Can you work these out from the model? Positions are in its coordinate system, mm. Face numbers are marked on the shaded views. A direction names the side the tool comes from. Coordinates: 2 decimals unless noted, no trailing zeros. Order: outer loops, then holes, each group sorted by start corner. A loop starts at its lowest first (then second) coordinate and runs counter-clockwise, first axis right, second up. Notation, with made-up numbers: (-6, -38.5) -> (14, -38.5) arc R18 cw to (14, -30.5) -> close; hole circle Ø7 at (62, 86.5). An arc over 180 degrees is marked (long way). Answer in a Markdown table with one row per item.
```python
from build123d import *

# Parameters (mm, degrees)
F0_W           = 50
F0_H           = 46
F0_R           = 11
F1_DEPTH       = 20
F2_W           = 44
F2_H           = 43
F3_DEPTH       = 17
F4_SIZE2       = 17
F4_SIZE        = 42
F5_D           = 3.1
F5_CSINK_D     = 6.72
F5_CSINK_ANGLE = 90
F6_T1_DEPTH    = 23.5734639037
F7_SIZE        = 1.5
F9_D           = 4.1
F9_CSINK_D     = 9
F9_CSINK_ANGLE = 90


# Not quite as in the source:
# - a fillet or chamfer that OpenCascade refuses, or shapes differently, is made with other operations: its cross-section is extruded or revolved along the edge and cut away or added


with BuildPart() as f1:
    # F0 (on Top) → F1 (new body)
    with BuildSketch(Plane.XY):
        with Locations((0, 2)):
            Rectangle(F0_W, F0_H)
        Circle(F0_R, mode=Mode.SUBTRACT)
    extrude(amount=-F1_DEPTH)

    # F2 (on face) → F3 (cut, through all)
    with BuildSketch(Plane(origin=(0, 0, -20), x_dir=(1, 0, 0), z_dir=(0, 0, -1))):
        with Locations((0, -0.5)):
            Rectangle(F2_W, F2_H)
    extrude(amount=-F3_DEPTH, mode=Mode.SUBTRACT)

    # F4
    f4_edges = [f1.edges().sort_by_distance(p)[0] for p in [
        (23.5, -21, -20),
        (-23.5, -21, -20),
    ]]
    f4_side = f1.faces().sort_by_distance((-24.320588, 2, -20))[0]
    chamfer(f4_edges, length=F4_SIZE, length2=F4_SIZE2, reference=f4_side)

    # F5 (through all)
    with Locations(Plane.XY):
        with Locations((15.5, 15.5), (-15.5, 15.5), (-15.5, -15.5), (15.5, -15.5)):
            CounterSinkHole(F5_D / 2, F5_CSINK_D / 2, counter_sink_angle=F5_CSINK_ANGLE)

    # F6: chamfer of 4 on 2 edges, made by hand

    # F6_s2 → F6_t1 (cut)
    with BuildSketch(Plane.XY.offset(-13.2867319519)):
        Polygon((-21, -21), (-25, -17), (-25, -21), align=None)
        Polygon((21, -21), (25, -17), (25, -21), align=None)
    extrude(amount=F6_T1_DEPTH, mode=Mode.SUBTRACT)

    # F7
    f7_edges = [f1.edges().sort_by_distance(p)[0] for p in [
        (-22, 22, -11.5),
        (22, 22, -11.5),
    ]]
    chamfer(f7_edges, length=F7_SIZE)

    # F9 (through all)
    with Locations(Plane.XZ.offset(-22)):
        with Locations((15, -10), (-15, -10)):
            CounterSinkHole(F9_D / 2, F9_CSINK_D / 2, counter_sink_angle=F9_CSINK_ANGLE)


solid = f1.part
```
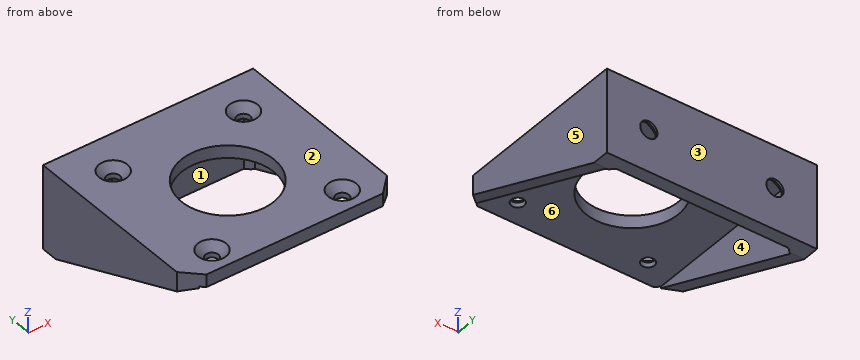
(1) Suppose I cut it at B-B (y = -2). Please give me the cut outline in (x, z), and give its area (3 significant figures).
Response values:
| item | result |
|---|---|
| outline | (-25, -10.69) -> (-22, -10.69) -> (-22, -3) -> (-10.82, -3) -> (-10.82, 0) -> (-25, 0) -> close; (10.82, -3) -> (22, -3) -> (22, -10.69) -> (25, -10.69) -> (25, 0) -> (10.82, 0) -> close |
| area | 131 mm2 |
(2) Suppose I cut it at A-A (x = 0). Please give me the cut outline in (y, z).
Response values:
| item | result |
|---|---|
| outline | (-21, -3) -> (-11, -3) -> (-11, 0) -> (-21, 0) -> close; (11, -3) -> (22, -3) -> (22, -20) -> (25, -20) -> (25, 0) -> (11, 0) -> close |
(3) Suppose I cut it at C-C (y = -15.5). Please give me the cut outline in (x, z), and give its area (3 significant figures).
Response values:
| item | result |
|---|---|
| outline | (-25, -5.23) -> (-22, -5.23) -> (-22, -3) -> (-17.05, -3) -> (-17.05, -1.81) -> (-18.86, 0) -> (-25, 0) -> close; (-13.95, -3) -> (13.95, -3) -> (13.95, -1.81) -> (12.14, 0) -> (-12.14, 0) -> (-13.95, -1.81) -> close; (17.05, -3) -> (22, -3) -> (22, -5.23) -> (25, -5.23) -> (25, 0) -> (18.86, 0) -> (17.05, -1.81) -> close |
| area | 138 mm2 |
(4) We'd pull the mould along X, two halves only. Please class the marked faces 3, 4, 5 and 6: +X half, -X half, draft (parallel to the pull), parting line (faces both ways), or undercut.
Response values:
| item | result |
|---|---|
| face 3 | draft |
| face 4 | undercut |
| face 5 | +X half |
| face 6 | undercut |
(5) On a 3-axis mill with a long thin cutter (end or side, diameter ignored), from which of +Z, -Z, +X, -X, +Y, -Y can I reach the whole of each face in a straight line? I mean the marked faces 1 and 2. Say none if no direction works.
Response values:
| item | result |
|---|---|
| face 1 | -Z, -Y |
| face 2 | +Z, +X, -X, +Y, -Y |
(6) Suppose I cut it at D-D (z = -10). Please give me the cut outline in (x, y).
Response values:
| item | result |
|---|---|
| outline | (-25, -3.71) -> (-22, -3.71) -> (-22, 20.5) -> (-20.5, 22) -> (-19.5, 22) -> (-17.05, 24.45) -> (-17.05, 25) -> (-25, 25) -> close; (-12.95, 24.45) -> (-10.5, 22) -> (10.5, 22) -> (12.95, 24.45) -> (12.95, 25) -> (-12.95, 25) -> close; (17.05, 24.45) -> (19.5, 22) -> (20.5, 22) -> (22, 20.5) -> (22, -3.71) -> (25, -3.71) -> (25, 25) -> (17.05, 25) -> close |
(7) Will these pins go through, and if not, where does the flat tip stop? pin 1 Ø3.5 at (x, y) = (15.5, 15.5) entering from +Z; pin 2 Ø4.5 at (x, z) = (15, -10) entering from -Y; pin 3 Ø13 at (x, y) = (0.5, 11) entering from -Z.
Response values:
| item | result |
|---|---|
| pin 1 | z = -1.61 |
| pin 2 | y = 24.25 |
| pin 3 | z = -3 |
(8) I need wall thicknesses on line 1 (Y direction, x = -15.5, z = -2.35); line 2 (X direction, y = -15.5, z = -2.35); line 3 (X direction, y = 11, z = -11.75). Which ranges of each line are inside material? Lowest first, please. Write a range as [from, to].
Response values:
| item | result |
|---|---|
| line 1 | [-21, -17.05], [-13.95, 13.95], [17.05, 25] |
| line 2 | [-25, -17.05], [-13.95, 13.95], [17.05, 25] |
| line 3 | [-25, -22], [22, 25] |
